Work out the finished part from the listing and answer in its coordinate system (mm). A direction names the side the tool comes from. Round coordinates to 2 decimals unless told otherwise and drop trailing zeros. Loops run counter-clockwise (first coordinate to the right, second up) from the corner with the lowest first, then second, coordinate; pieces in that order, holes last. Notation, with made-up numbers: M -29.5,57 L -8.5,57 A5 ccw -8.5,62 Z; hole C 54.5,-19.5 d1. An arc over 180 degrees is marked long. One line per item, written item: value.
```python
from build123d import *

# Parameters (mm, degrees)
F0_W     = 142
F0_H     = 177
F1_DEPTH = 20
F2_W     = 138
F2_H     = 173
F3_DEPTH = 18
F4_DEPTH = 9
F5_W     = 157
F5_H     = 10
F6_DEPTH = 10
F7_R     = 2


with BuildPart() as f1:
    # F0 (on Top) → F1 (new body)
    with BuildSketch(Plane.XY):
        with Locations((10.088578, 15.472607)):
            Rectangle(F0_W, F0_H)
    extrude(amount=F1_DEPTH)

    # F2 (on face) → F3 (cut)
    with BuildSketch(Plane.XY.offset(20)):
        with Locations((10.088578, 15.472607)):
            Rectangle(F2_W, F2_H)
    extrude(amount=-F3_DEPTH, mode=Mode.SUBTRACT)

    # F2 (on face) → F4 (cut)
    with BuildSketch(Plane.XY.offset(20)):
        Polygon((-60.911422, -73.027393), (79.088578, -73.027393), (79.088578, -71.027393), (-58.911422, -71.027393), (-58.911422, 101.972607), (79.088578, 101.972607), (79.088578, 103.972607), (-60.911422, 103.972607), align=None)
    extrude(amount=-F4_DEPTH, mode=Mode.SUBTRACT)

    # F5 (on face) → F6 (join)
    with BuildSketch(Plane.YZ.offset(81.088578)):
        with Locations((15.472607, 10)):
            Rectangle(F5_W, F5_H)
    extrude(amount=F6_DEPTH)

    # F7
    f7_edges = [f1.edges().sort_by_distance(p)[0] for p in [
        (91.088578, 15.472607, 15),
        (91.088578, 15.472607, 5),
        (91.088578, -63.027393, 10),
        (91.088578, 93.972607, 10),
    ]]
    fillet(f7_edges, radius=F7_R)


solid = f1.part
```
1) Each of these flat-tipped pins is pushed along its axis until it touches: pin 1 (1.5 mm diameter, centred on x = 14.5, y = 62.5, fed in from +Z); pin 2 (6.5 mm diameter, centred on x = 84, y = -16, fed in from -Z); pin 3 (6.5 mm diameter, centred on x = 84.5, z = 10.5, fed in from -Y); pin 4 (4 mm diameter, centred on x = 85, y = -9, fed in from +Z). Where does it stop, or does it pass through?
Check values:
pin 1: z = 2
pin 2: z = 0
pin 3: y = -63.03
pin 4: z = 15
2) Find section A-A (y = -54). Give the vertices of the cut face in (x, z), then the cut area to 3 significant figures.
Check values:
outline: M -60.91,0 L 81.09,0 L 81.09,5 L 89.09,5 A2 ccw 91.09,7 L 91.09,13 A2 ccw 89.09,15 L 81.09,15 L 81.09,20 L 79.09,20 L 79.09,2 L -58.91,2 L -58.91,11 L -60.91,11 Z
area: 436 mm2
3) Find section B-B (x = 30.5). Give the vertices of the cut face in (y, z), then the cut area to 3 significant figures.
Check values:
outline: M -73.03,0 L 103.97,0 L 103.97,11 L 101.97,11 L 101.97,2 L -71.03,2 L -71.03,11 L -73.03,11 Z
area: 390 mm2
4) Find the intervals of material crossed by probe 1 along X at (y, z) = (6, 2.75); probe 2 along Y at (x, z) = (55.5, 10.75); probe 3 along Z at (x, y) = (71.5, 31), in increasing order. Write a range as from..to.
Check values:
probe 1: -60.91..-58.91, 79.09..81.09
probe 2: -73.03..-71.03, 101.97..103.97
probe 3: 0..2
5) For faces 4 (the face through (85, 93.973, 10)), 5 (the face through (85, -63.027, 10)), 6 (the face through (9, 17, 2)), determine the directions among +Z, -Z, +X, -X, +Y, -Y from which every point of the face is accessible in a straight line to the end or side of a thin tool.
Check values:
face 4: +Z, -Z, +X, +Y
face 5: +Z, -Z, +X, -Y
face 6: +Z
6) The mould has two halves that part along X. Classify faces 1 (the face through (9, 103.973, 5)), 2 (the face through (79.089, 14, 11)), 3 (the face through (91.089, 14, 10)): +X half, -X half, draft (parallel to the pull), parting line (faces both ways), or undercut.
Check values:
face 1: draft
face 2: undercut
face 3: +X half
